Here's how the part is built. I have some questions about the finished solid (model axes, mm). A direction names the side the tool comes from. Round coordinates to 2 decimals unless told otherwise and drop trailing zeros. Order: outer loops, then holes, each group sorted by start corner. A loop starts at its lowest first (then second) coordinate and runs counter-clockwise, first axis right, second up. Notation, with made-up numbers: (-5, 76.5) -> (5, 76.5) arc R18 ccw to (5, 105.5) -> close; hole circle Ø4 at (-6.5, -22). An arc over 180 degrees is marked (long way). One line per item, written item: value.
```python
from build123d import *

# Parameters (mm, degrees)
SKETCH_W        = 12
SKETCH_H        = 4
PAD_DEPTH       = 76
POCKET_START    = -7
SKETCH001_R     = 6.05
POCKET_DEPTH    = 62
SKETCH002_R     = 5.05
POCKET001_DEPTH = 76.001
SKETCH003_W     = 12
SKETCH003_H     = 62
POCKET002_DEPTH = 2
SKETCH004_W     = 4
SKETCH004_H     = 62
POCKET003_DEPTH = 2.001
SKETCH005_W     = 12
SKETCH005_H     = 14
PAD001_DEPTH    = 2
SKETCH006_W     = 8
SKETCH006_H     = 14
POCKET004_DEPTH = 5
SKETCH007_R     = 1
POCKET005_DEPTH = 4.001
FILLET_R        = 1
FILLET001_R     = 1
FILLET002_R     = 1
FILLET003_R     = 1
FILLET004_R     = 1
FILLET005_R     = 1
FILLET006_R     = 1
FILLET007_R     = 1
FILLET008_R     = 1
FILLET009_R     = 1
FILLET010_R     = 1


with BuildPart() as part:
    # Sketch → Pad (new body)
    with BuildSketch(Plane.YZ):
        with Locations((6, 2)):
            Rectangle(SKETCH_W, SKETCH_H)
    extrude(amount=PAD_DEPTH)

    # Sketch001 (on Face6 of Pad) → Pocket (cut)
    with BuildSketch(Plane.YZ.offset(76).offset(POCKET_START)):
        with Locations((6, 8)):
            Circle(SKETCH001_R)
    extrude(amount=-POCKET_DEPTH, mode=Mode.SUBTRACT)

    # Sketch002 (on Face5 of Pocket) → Pocket001 (cut, through all)
    with BuildSketch(Plane.YZ.offset(76)):
        with Locations((6, 8)):
            Circle(SKETCH002_R)
    extrude(amount=-POCKET001_DEPTH, mode=Mode.SUBTRACT)

    # Sketch003 (on Face1 of Pocket001) → Pocket002 (cut)
    with BuildSketch(Plane.YX):
        with Locations((6, 38)):
            Rectangle(SKETCH003_W, SKETCH003_H)
    extrude(amount=-POCKET002_DEPTH, mode=Mode.SUBTRACT)

    # Sketch004 (on Face12 of Pocket002) → Pocket003 (cut, through all)
    with BuildSketch(Plane.YX.offset(-2)):
        with Locations((6, 38)):
            Rectangle(SKETCH004_W, SKETCH004_H)
    extrude(amount=-POCKET003_DEPTH, mode=Mode.SUBTRACT)

    # Sketch005 (on Face12 of Pocket003) → Pad001 (join)
    with BuildSketch(Plane.YX.offset(-2)):
        with Locations((6, 38)):
            Rectangle(SKETCH005_W, SKETCH005_H)
    extrude(amount=PAD001_DEPTH)

    # Sketch006 (on Face35 of Pad001) → Pocket004 (cut)
    with BuildSketch(Plane.YX):
        with Locations((6, 38)):
            Rectangle(SKETCH006_W, SKETCH006_H)
    extrude(amount=-POCKET004_DEPTH, mode=Mode.SUBTRACT)

    # Sketch007 (on Face10 of Pocket004) → Pocket005 (cut, through all)
    with BuildSketch(Plane.YX):
        with Locations((6, 3.5)):
            Circle(SKETCH007_R)
        with Locations((6, 72.5)):
            Circle(SKETCH007_R)
    extrude(amount=-POCKET005_DEPTH, mode=Mode.SUBTRACT)

    # Fillet
    fillet_edges = [part.edges().sort_by_distance(p)[0] for p in [
        (45, 11, 2),
    ]]
    fillet(fillet_edges, radius=FILLET_R)

    # Fillet001
    fillet001_edges = [part.edges().sort_by_distance(p)[0] for p in [
        (31, 11, 2),
    ]]
    fillet(fillet001_edges, radius=FILLET001_R)

    # Fillet002
    fillet002_edges = [part.edges().sort_by_distance(p)[0] for p in [
        (31, 1, 2),
    ]]
    fillet(fillet002_edges, radius=FILLET002_R)

    # Fillet003
    fillet003_edges = [part.edges().sort_by_distance(p)[0] for p in [
        (45, 1, 2),
    ]]
    fillet(fillet003_edges, radius=FILLET003_R)

    # Fillet004
    fillet004_edges = [part.edges().sort_by_distance(p)[0] for p in [
        (69, 10, 2),
    ]]
    fillet(fillet004_edges, radius=FILLET004_R)

    # Fillet005
    fillet005_edges = [part.edges().sort_by_distance(p)[0] for p in [
        (69, 2, 2),
    ]]
    fillet(fillet005_edges, radius=FILLET005_R)

    # Fillet006
    fillet006_edges = [part.edges().sort_by_distance(p)[0] for p in [
        (7, 10, 2),
    ]]
    fillet(fillet006_edges, radius=FILLET006_R)

    # Fillet007
    fillet007_edges = [part.edges().sort_by_distance(p)[0] for p in [
        (31, 10, 2.730501),
    ]]
    fillet(fillet007_edges, radius=FILLET007_R)

    # Fillet008
    fillet008_edges = [part.edges().sort_by_distance(p)[0] for p in [
        (45, 10, 2.730501),
    ]]
    fillet(fillet008_edges, radius=FILLET008_R)

    # Fillet009
    fillet009_edges = [part.edges().sort_by_distance(p)[0] for p in [
        (31, 2, 2.730501),
    ]]
    fillet(fillet009_edges, radius=FILLET009_R)

    # Fillet010
    fillet010_edges = [part.edges().sort_by_distance(p)[0] for p in [
        (45, 2, 2.730501),
    ]]
    fillet(fillet010_edges, radius=FILLET010_R)


solid = part.part
```
Q1. Which directions (+Z, -Z, +X, -X, +Y, -Y) give clear straight access to the entire face, cutting with the end or side of a thin tool? Please do faces 1 (the face through (38.434, 1.802, 3.643)), 2 (the face through (7, 5, 2)), 3 (the face through (71.61, 6.46, 1.5)).
Answers:
face 1: +Z
face 2: none
face 3: +Z, -Z
Q2. I want a section at B-B on y = 6. Write out the boundary of the cut face in (x, z), then the cut area to 3 significant figures.
Answers:
outline: (0, 0) -> (2.5, 0) -> (2.5, 2.95) -> (0, 2.95) -> close; (4.5, 0) -> (7, 0) -> (7, 2.95) -> (4.5, 2.95) -> close; (69, 0) -> (71.5, 0) -> (71.5, 2.95) -> (69, 2.95) -> close; (73.5, 0) -> (76, 0) -> (76, 2.95) -> (73.5, 2.95) -> close
area: 29.5 mm2
Q3. For P1, Ø0.6, axis at y = 8.5, z = 2, coming from the -X side; P2, Ø1.6, axis at x = 3.5, y = 6, coming from the -Z side; P3, Ø4, axis at x = 64, y = 7, coming from the +Z side; P4, Ø1.2, axis at x = 59, y = 10.5, coming from the -Z side, each with a flat end and sliding along its axis, tell me the tip position at first contact or that it passes through.
Answers:
P1: x = 0
P2: through
P3: z = 2.75
P4: z = 2
Q4. I want a section at C-C on x = 60.5. Write out the boundary of the cut face in (y, z).
Answers:
outline: (0, 2) -> (4, 2) -> (4, 2.29) arc R6.05 cw to (1.46, 4) -> (0, 4) -> close; (8, 2) -> (12, 2) -> (12, 4) -> (10.54, 4) arc R6.05 cw to (8, 2.29) -> close
Q5. I want a section at A-A on x = 3.5. Write out the boundary of the cut face in (y, z), then the cut area to 3 significant figures.
Answers:
outline: (0, 0) -> (5, 0) -> (5, 3.05) arc R5.05 cw to (2.92, 4) -> (0, 4) -> close; (7, 0) -> (12, 0) -> (12, 4) -> (9.08, 4) arc R5.05 cw to (7, 3.05) -> close
area: 37.6 mm2
Q6. I need wall thicknesses on line 1 along X through (y, z) = (6, 2.4); line 2 along Y through (x, z) = (72.5, 1.9); line 3 along Y through (x, z) = (41, 2.9). Which ranges of each line are inside material? Lowest first, please.
Answers:
line 1: 0 to 2.5, 4.5 to 7, 69 to 71.5, 73.5 to 76
line 2: 0 to 5, 7 to 12
line 3: 0 to 2, 10 to 12
Q7. If we mould it in two halves opening along X, with no side actions, what happens to faces 4 (the face through (76, 6, 2)), 5 (the face through (69, 6, 2)), 6 (the face through (72.5, 4.6, 0))? For each: pulls with the +X half, pulls with the -X half, needs draft (parallel to the pull), parting line crosses it, or undercut.
Answers:
face 4: pulls with the +X half
face 5: undercut
face 6: needs draft
